from build123d import *

# Parameters (mm, degrees)
SKETCH_1_W      = 86
SKETCH_1_H      = 86
EXTRUDE_2_DEPTH = 10
SKETCH_2_W      = 32
SKETCH_2_H      = 56
EXTRUDE_3_DEPTH = 5.5


with BuildPart() as part:
    # 草图1 → 凸台-拉伸2 (new body)
    with BuildSketch(Plane.XY):
        Rectangle(SKETCH_1_W, SKETCH_1_H)
    extrude(amount=-EXTRUDE_2_DEPTH)

    # 草图2 → 凸台-拉伸3 (add)
    with BuildSketch(Plane.XY):
        with Locations((17, -5)):
            Rectangle(SKETCH_2_W, SKETCH_2_H)
        with Locations((-16, -5)):
            Rectangle(SKETCH_2_W, SKETCH_2_H)
    extrude(amount=EXTRUDE_3_DEPTH)


solid = part.part
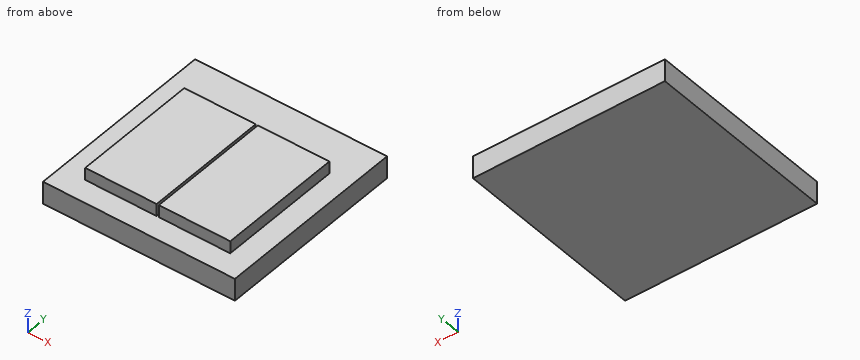
The listing builds one solid part. Answer for the finished solid, in the listing's coordinates (mm). Give positions to 0.01 mm unless a question says otherwise; leave off trailing zeros. Write each loop counter-clockwise with the first axis right and the second up, starting at its lowest first coordinate (ties: lowest second). Pieces come first, ordered by that corner, then holes. Notation, with made-up numbers: (56.5, 34.25) -> (60.5, 34.25) arc R7 ccw to (60.5, 44.25) -> close; hole circle Ø10 at (27, 79). An arc over 180 degrees is marked (long way). Use a Markdown table: item, result.
(1) Section A-A, the plane z = 4.25 is taken. Determine the outline of the cut face in (x, y), then the cut area to 3 significant figures.
Return value:
| item | result |
|---|---|
| outline | (-32, -33) -> (0, -33) -> (0, 23) -> (-32, 23) -> close; (1, -33) -> (33, -33) -> (33, 23) -> (1, 23) -> close |
| area | 3,580 mm2 |
(2) Flat-ended cylindrical pins translate along their axes: P1, Ø1.6, axis at y = -9.5, z = 3, coming from the +X side; P2, Ø6, axis at y = -18, z = 3.5, coming from the -X side; P3, Ø3, axis at x = 19.5, z = 4, coming from the -Y side; P4, Ø2, axis at y = 28, z = 2.5, coming from the +X side. Find the tip coordinate at first contact, or state that the pin passes through.
Return value:
| item | result |
|---|---|
| P1 | x = 33 |
| P2 | x = -32 |
| P3 | y = -33 |
| P4 | through |
(3) Section D-D, the plane y = 36 is taken. Determine the outline of the cut face in (x, z).
Return value:
| item | result |
|---|---|
| outline | (-43, -10) -> (43, -10) -> (43, 0) -> (-43, 0) -> close |
(4) Section C-C, the plane x = 12.5 is taken. Determine the outline of the cut face in (y, z).
Return value:
| item | result |
|---|---|
| outline | (-43, -10) -> (43, -10) -> (43, 0) -> (23, 0) -> (23, 5.5) -> (-33, 5.5) -> (-33, 0) -> (-43, 0) -> close |
(5) Section B-B, the plane y = -23.5 is taken. Determine the outline of the cut face in (x, z).
Return value:
| item | result |
|---|---|
| outline | (-43, -10) -> (43, -10) -> (43, 0) -> (33, 0) -> (33, 5.5) -> (1, 5.5) -> (1, 0) -> (0, 0) -> (0, 5.5) -> (-32, 5.5) -> (-32, 0) -> (-43, 0) -> close |
(6) Find the intervals of material crossed by probe 1 along X at (y, z) = (2, 2.5); probe 2 along Z at (x, y) = (-29, -36.5); probe 3 along Y at (x, z) = (30.5, 1.5), in increasing order. Write a range as from..to.
Return value:
| item | result |
|---|---|
| probe 1 | -32..0, 1..33 |
| probe 2 | -10..0 |
| probe 3 | -33..23 |
